Read the model definition and answer for the solid it produces. Units are mm, in the model's axes. A direction names the side the tool comes from. Give positions to 0.01 mm unless a question says otherwise; leave off trailing zeros. Write each loop counter-clockwise with the first axis right and the second up, starting at its lowest first coordinate (ties: lowest second). Pieces come first, ordered by that corner, then holes. Notation, with made-up numbers: (-16.75, -34.75) - (32.25, -34.75) arc R17 cw to (32.25, -19.75) - close; hole circle Ø6 at (-11.75, 27.5). An arc over 180 degrees is marked (long way). Answer as a JSON object with one key per item and string values. Group by question number.
```python
from build123d import *

# Parameters (mm, degrees)
EXTRUDE_1_DEPTH          = 2
HOLE_WIZARD_1_D          = 2.5
CUT_EXTRUDE_1_DEPTH      = 71.244216844
EXTRUDE_2_DEPTH          = 2
CUT_EXTRUDE_2_DEPTH      = 71.244216844
CUT_EXTRUDE_2_DEPTH_BACK = 71.244216844
EXTRUDE_3_DEPTH          = 2
CUT_EXTRUDE_3_DEPTH      = 72.517917335
CUT_EXTRUDE_3_DEPTH_BACK = 72.517917335
EXTRUDE_4_DEPTH          = 2
HOLE_WIZARD_2_D          = 2.5


with BuildPart() as part:
    # 草图1 → 凸台-拉伸1 (new body)
    with BuildSketch(Plane(origin=(0, 0, 0), x_dir=(1, 0, 0), z_dir=(0, 1, 0))):
        with BuildLine():
            Line((66.5, 10), (-66.5, 10))
            ThreePointArc((-66.5, 10), (-68.621320344, 9.121320344), (-69.5, 7))
            Line((-69.5, 7), (-69.5, -7))
            ThreePointArc((-69.5, -7), (-68.621320344, -9.121320344), (-66.5, -10))
            Line((-66.5, -10), (66.5, -10))
            ThreePointArc((66.5, -10), (68.621320344, -9.121320344), (69.5, -7))
            Line((69.5, -7), (69.5, 7))
            ThreePointArc((69.5, 7), (68.621320344, 9.121320344), (66.5, 10))
        make_face()
    extrude(amount=EXTRUDE_1_DEPTH)

    # 孔1 (through all)
    with Locations(Plane(origin=(0, 2, 0), x_dir=(1, 0, 0), z_dir=(0, 1, 0))):
        with Locations((-64.5, 6), (-64.5, -6), (64.5, -6), (64.5, 6)):
            Hole(HOLE_WIZARD_1_D / 2)

    # 草图5 → 切除-拉伸1 (cut, through all)
    with BuildSketch(Plane(origin=(0, 2, 0), x_dir=(1, 0, 0), z_dir=(0, 1, 0))):
        with BuildLine():
            Line((-54.5, 7), (54.5, 7))
            ThreePointArc((54.5, 7), (61.5, 0), (54.5, -7))
            Line((54.5, -7), (-54.5, -7))
            ThreePointArc((-54.5, -7), (-61.5, 0), (-54.5, 7))
        make_face()
    extrude(amount=-CUT_EXTRUDE_1_DEPTH, mode=Mode.SUBTRACT)

    # 草图6 → 凸台-拉伸2 (add)
    with BuildSketch(Plane.XZ):
        with BuildLine():
            Line((-39.249952973, -9.999988019), (39.249952973, -9.999988019))
            Line((39.249952973, -9.999988019), (46.785993788, -7))
            Line((46.785993788, -7), (42.25, -7))
            ThreePointArc((42.25, -7), (40.128679656, -6.121320344), (39.25, -4))
            Line((39.25, -4), (39.25, 4))
            ThreePointArc((39.25, 4), (40.128679656, 6.121320344), (42.25, 7))
            Line((42.25, 7), (46.785993788, 7))
            Line((46.785993788, 7), (39.25, 10))
            Line((39.25, 10), (-39.25, 10))
            Line((-39.25, 10), (-46.786070913, 7))
            Line((-46.786070913, 7), (-42.25, 7))
            ThreePointArc((-42.25, 7), (-40.128679656, 6.121320344), (-39.25, 4))
            Line((-39.25, 4), (-39.25, -4))
            ThreePointArc((-39.25, -4), (-40.128679656, -6.121320344), (-42.25, -7))
            Line((-42.25, -7), (-46.49444439, -7))
            Line((-46.49444439, -7), (-39.249952973, -9.999988019))
        make_face()
    extrude(amount=-EXTRUDE_2_DEPTH)

    # 草图7 → 切除-拉伸2 (cut, two sides: drawn at the far end of the back side and taken through both)
    with BuildSketch(Plane.XZ.offset(-CUT_EXTRUDE_2_DEPTH_BACK)):
        with BuildLine():
            Line((34.25, -1.5), (-34.25, -1.5))
            ThreePointArc((-34.25, -1.5), (-35.75, 0), (-34.25, 1.5))
            Line((-34.25, 1.5), (34.25, 1.5))
            ThreePointArc((34.25, 1.5), (35.75, 0), (34.25, -1.5))
        make_face()
        with BuildLine():
            Line((34.25, 4), (-34.25, 4))
            ThreePointArc((-34.25, 4), (-35.75, 5.5), (-34.25, 7))
            Line((-34.25, 7), (34.25, 7))
            ThreePointArc((34.25, 7), (35.75, 5.5), (34.25, 4))
        make_face()
        with BuildLine():
            Line((34.25, -7), (-34.25, -7))
            ThreePointArc((-34.25, -7), (-35.75, -5.5), (-34.25, -4))
            Line((-34.25, -4), (34.25, -4))
            ThreePointArc((34.25, -4), (35.75, -5.5), (34.25, -7))
        make_face()
    extrude(amount=CUT_EXTRUDE_2_DEPTH + CUT_EXTRUDE_2_DEPTH_BACK, mode=Mode.SUBTRACT)

    # 草图9 → 凸台-拉伸3 (add)
    with BuildSketch(Plane(origin=(0, 0, 0), x_dir=(-1, 0, 0), z_dir=(0, -1, 0))):
        with BuildLine():
            ThreePointArc((37.785533906, -11.464466094), (39.40765065, -10.380602337), (41.321067812, -10))
            Line((41.321067812, -10), (39.25, -10))
            Line((39.25, -10), (33.593145751, -10))
            Line((33.593145751, -10), (32.307611845, -11.285533906))
            ThreePointArc((32.307611845, -11.285533906), (30.6854951, -12.369397663), (28.772077939, -12.75))
            Line((28.772077939, -12.75), (-28.772077939, -12.75))
            ThreePointArc((-28.772077939, -12.75), (-30.6854951, -12.369397663), (-32.307611845, -11.285533906))
            Line((-32.307611845, -11.285533906), (-33.593145751, -10))
            Line((-33.593145751, -10), (-39.25, -10))
            Line((-39.25, -10), (-41.321067812, -10))
            ThreePointArc((-41.321067812, -10), (-39.40765065, -10.380602337), (-37.785533906, -11.464466094))
            Line((-37.785533906, -11.464466094), (-33.964466094, -15.285533906))
            ThreePointArc((-33.964466094, -15.285533906), (-32.34234935, -16.369397663), (-30.428932188, -16.75))
            Line((-30.428932188, -16.75), (30.428932188, -16.75))
            ThreePointArc((30.428932188, -16.75), (32.34234935, -16.369397663), (33.964466094, -15.285533906))
            Line((33.964466094, -15.285533906), (37.785533906, -11.464466094))
        make_face()
        with BuildLine():
            Line((32.307611845, 11.285533906), (33.593145751, 10))
            Line((33.593145751, 10), (39.25, 10))
            Line((39.25, 10), (41.321067812, 10))
            ThreePointArc((41.321067812, 10), (39.40765065, 10.380602337), (37.785533906, 11.464466094))
            Line((37.785533906, 11.464466094), (33.964466094, 15.285533906))
            ThreePointArc((33.964466094, 15.285533906), (32.34234935, 16.369397663), (30.428932188, 16.75))
            Line((30.428932188, 16.75), (-30.428932188, 16.75))
            ThreePointArc((-30.428932188, 16.75), (-32.34234935, 16.369397663), (-33.964466094, 15.285533906))
            Line((-33.964466094, 15.285533906), (-37.785533906, 11.464466094))
            ThreePointArc((-37.785533906, 11.464466094), (-39.40765065, 10.380602337), (-41.321067812, 10))
            Line((-41.321067812, 10), (-39.25, 10))
            Line((-39.25, 10), (-33.593145751, 10))
            Line((-33.593145751, 10), (-32.307611845, 11.285533906))
            ThreePointArc((-32.307611845, 11.285533906), (-30.6854951, 12.369397663), (-28.772077939, 12.75))
            Line((-28.772077939, 12.75), (28.772077939, 12.75))
            ThreePointArc((28.772077939, 12.75), (30.6854951, 12.369397663), (32.307611845, 11.285533906))
        make_face()
    extrude(amount=-EXTRUDE_3_DEPTH)

    # 草图10 → 切除-拉伸3 (cut, two sides: drawn at the far end of the back side and taken through both)
    with BuildSketch(Plane(origin=(0, 2, 0), x_dir=(1, 0, 0), z_dir=(0, 1, 0)).offset(-CUT_EXTRUDE_3_DEPTH_BACK)):
        with BuildLine():
            Line((34.285533906, -9.307611845), (34.098025299, -9.495120452))
            ThreePointArc((34.098025299, -9.495120452), (32.487874075, -10.574009752), (30.588407989, -10.959519378))
            Line((30.588407989, -10.959519378), (-30.221374051, -11.274720124))
            ThreePointArc((-30.221374051, -11.274720124), (-32.148729436, -10.899128383), (-33.782824553, -9.810321198))
            Line((-33.782824553, -9.810321198), (-34.285533906, -9.307611845))
            ThreePointArc((-34.285533906, -9.307611845), (-35.369397663, -7.6854951), (-35.75, -5.772077939))
            Line((-35.75, -5.772077939), (-35.75, 5.772077939))
            ThreePointArc((-35.75, 5.772077939), (-35.369397663, 7.6854951), (-34.285533906, 9.307611845))
            Line((-34.285533906, 9.307611845), (-33.772077939, 9.821067812))
            ThreePointArc((-33.772077939, 9.821067812), (-32.149961195, 10.904931568), (-30.236544033, 11.285533906))
            Line((-30.236544033, 11.285533906), (30.236544033, 11.285533906))
            ThreePointArc((30.236544033, 11.285533906), (32.149961195, 10.904931568), (33.772077939, 9.821067812))
            Line((33.772077939, 9.821067812), (34.285533906, 9.307611845))
            ThreePointArc((34.285533906, 9.307611845), (35.369397663, 7.6854951), (35.75, 5.772077939))
            Line((35.75, 5.772077939), (35.75, -5.772077939))
            ThreePointArc((35.75, -5.772077939), (35.369397663, -7.6854951), (34.285533906, -9.307611845))
        make_face()
    extrude(amount=CUT_EXTRUDE_3_DEPTH + CUT_EXTRUDE_3_DEPTH_BACK, mode=Mode.SUBTRACT)

    # 草图11 → 凸台-拉伸4 (add)
    with BuildSketch(Plane.XZ):
        with BuildLine():
            Line((-70, -10.165525061), (-70, -33.822863961))
            Line((-70, -33.822863961), (-60, -33.822863961))
            Line((-60, -33.822863961), (-31.125084611, -17.151923789))
            ThreePointArc((-31.125084611, -17.151923789), (-30.401541746, -16.852222521), (-29.625084611, -16.75))
            Line((-29.625084611, -16.75), (-21.789130896, -16.75))
            Line((-21.789130896, -16.75), (-32.229816093, -13.630777579))
            Line((-32.229816093, -13.630777579), (-39.940851874, -9.309148126))
            Line((-39.940851874, -9.309148126), (-37.434698294, -11.815301706))
            ThreePointArc((-37.434698294, -11.815301706), (-36.581684053, -14.328200626), (-38.056018637, -16.534698261))
            Line((-38.056018637, -16.534698261), (-55.5, -26.605985597))
            ThreePointArc((-55.5, -26.605985597), (-58.5, -26.605985597), (-60, -24.007909385))
            Line((-60, -24.007909385), (-60, -13))
            ThreePointArc((-60, -13), (-59.121320344, -10.878679656), (-57, -10))
            Line((-57, -10), (-53.184301675, -10))
            Line((-53.184301675, -10), (-53.184301675, -8.509493359))
            Line((-53.184301675, -8.509493359), (-68.301691744, -8.509493359))
            Line((-68.301691744, -8.509493359), (-69.5, -3.184578382))
            Line((-69.5, -3.184578382), (-69.5, -6.834474939))
            ThreePointArc((-69.5, -6.834474939), (-69.506814648, -6.999436002), (-69.527212152, -7.163272914))
            Line((-69.527212152, -7.163272914), (-69.972787848, -9.836727086))
            ThreePointArc((-69.972787848, -9.836727086), (-69.993185352, -10.000563998), (-70, -10.165525061))
        make_face()
        with BuildLine():
            Line((68.301691744, -8.509493359), (69.5, -3.534682622))
            Line((69.5, -3.534682622), (69.5, -6.834474939))
            ThreePointArc((69.5, -6.834474939), (69.506814648, -6.999436002), (69.527212152, -7.163272914))
            Line((69.527212152, -7.163272914), (69.972787848, -9.836727086))
            ThreePointArc((69.972787848, -9.836727086), (69.993185352, -10.000563998), (70, -10.165525061))
            Line((70, -10.165525061), (70, -33.822863961))
            Line((70, -33.822863961), (60, -33.822863961))
            Line((60, -33.822863961), (31.125084611, -17.151923789))
            ThreePointArc((31.125084611, -17.151923789), (30.401541746, -16.852222521), (29.625084611, -16.75))
            Line((29.625084611, -16.75), (21.789130896, -16.75))
            Line((21.789130896, -16.75), (32.229816093, -13.630777579))
            Line((32.229816093, -13.630777579), (39.940851874, -9.309148126))
            Line((39.940851874, -9.309148126), (37.434698294, -11.815301706))
            ThreePointArc((37.434698294, -11.815301706), (36.581684053, -14.328200626), (38.056018637, -16.534698261))
            Line((38.056018637, -16.534698261), (55.5, -26.605985597))
            ThreePointArc((55.5, -26.605985597), (58.5, -26.605985597), (60, -24.007909385))
            Line((60, -24.007909385), (60, -13))
            ThreePointArc((60, -13), (59.121320344, -10.878679656), (57, -10))
            Line((57, -10), (53.184301675, -10))
            Line((53.184301675, -10), (53.184301675, -8.509493359))
            Line((53.184301675, -8.509493359), (68.301691744, -8.509493359))
        make_face()
    extrude(amount=-EXTRUDE_4_DEPTH)

    # 孔2 (through all)
    with Locations(Plane(origin=(0, 0, 0), x_dir=(-1, 0, 0), z_dir=(0, -1, 0))):
        with Locations((65, 15.822863961), (65, 28.822863961), (-65, 15.822863961), (-65, 28.822863961)):
            Hole(HOLE_WIZARD_2_D / 2)


solid = part.part
```
1) Find section C-C, the plane y = 1.15. Give the number of separate pieces and of enclosed holes in the cut face, and give its area (3 significant figures).
2) For a pull along Z with two mould halves and no side action, classify faces 1 (the cylindrical face through (-68.64, 0.99, 9.1)), 2 (the flat face through (-45.76, 0.99, -25.6)), 3 (the flat face through (-1, 0, -14)), 4 (the cylindrical face through (-63.81, 1.01, -29.2)) as released by +Z, released by -Z, zero draft, split by the parting line, or undercut.
3) Which of the six approach directions +Z, -Z, +X, -X, +Y, -Y give full straight-line access (tool end or side, diameter ignored) to faces 5 (the flat face through (35.9, 0.99, 13.35)), 6 (the cylindrical face through (-58.46, 0.99, -26.63))?
4) Find section B-B, the plane z = 0.5. Write down the section's boundary in (x, y).
5) Flat-ended cylindrical pins translate along their axes: pin 1 Ø1 at (y, z) = (1, 1) entering from +X; pin 2 Ø2 at (x, z) = (-64.5, 6) entering from +Y; pin 3 Ø3 at (x, z) = (65, -15.82) entering from -Y. Find the tip coordinate at first contact, or state that the pin passes through.
6) Find section A-A, the plane x = 11. Write down the section's boundary in (y, z).
7) Find the intervals of material crossed by line 1 (Z direction, x = -55, y = 1); line 2 (Z direction, x = 20, y = 0.25); line 3 (X direction, y = 1.6, z = -17.5), in increasing order. Write a range as [from, to].
Values follow:
{
 "1": {"separate pieces": "1", "enclosed holes": "13", "area": "2,110 mm2"},
 "2": {"face 1": "released by +Z", "face 2": "released by -Z", "face 3": "zero draft", "face 4": "undercut"},
 "3": {"face 5": "+Z, +X, +Y, -Y", "face 6": "+Y, -Y"},
 "4": {"outline": "(-69.5, 0) - (-61.48, 0) - (-61.48, 2) - (-69.5, 2) - close; (-39.25, 0) - (-35.75, 0) - (-35.75, 2) - (-39.25, 2) - close; (35.75, 0) - (39.25, 0) - (39.25, 2) - (35.75, 2) - close; (61.48, 0) - (69.5, 0) - (69.5, 2) - (61.48, 2) - close"},
 "5": {"pin 1": "stops at x = 69.5", "pin 2": "passes through", "pin 3": "stops at y = 0"},
 "6": {"outline": "(0, -16.75) - (2, -16.75) - (2, -12.75) - (0, -12.75) - close; (0, 12.75) - (2, 12.75) - (2, 16.75) - (0, 16.75) - close"},
 "7": {"line 1": "z = [-30.94, -26.32], [-10, -6.98], [6.98, 10]", "line 2": "z = [-16.75, -12.75], [12.75, 16.75]", "line 3": "x = [-70, -60], [-39.73, -31.73], [31.73, 39.73], [60, 70]"}
}
